Verification items for this drawing (mm, ordinates from the low corner). A direction names the side the tool comes from. Round coordinates to 2 decimals unless told otherwise and drop trailing zeros. Loops run counter-clockwise (first coordinate to the right, second up) from the corner with the lowest first, then second, coordinate; pieces in that order, holes last. Notation, with made-up numbers: (42, -17) - (51, -17) arc R5 cw to (51, -12) - close; hole circle Ø6 at (89, 81). An arc over 180 degrees is marked (long way). Put each result on its own line as item: value.
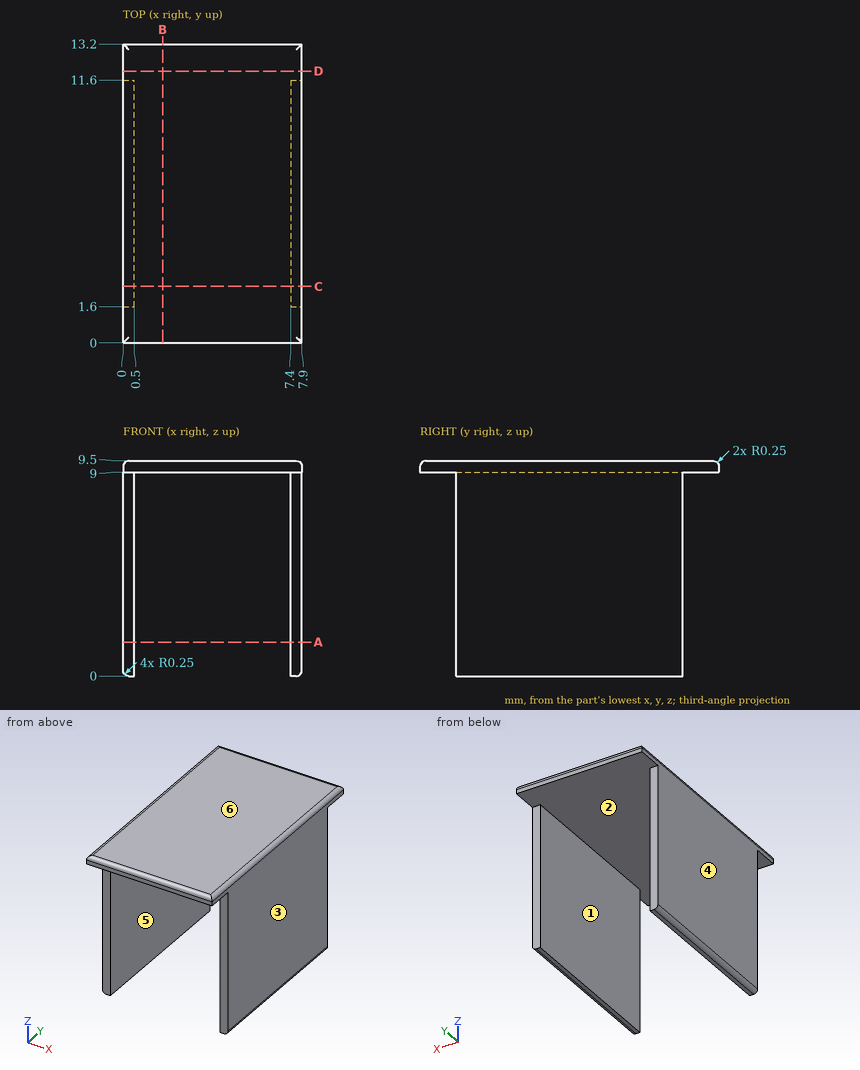
Item 1: Section check C-C on y = 2.5. Enter the section's corners in (x, z), then the cut area to 3 significant figures.
Filled sheet:
outline: (0, 0.25) arc R0.25 ccw to (0.25, 0) - (0.5, 0) - (0.5, 9) - (7.4, 9) - (7.4, 0) - (7.65, 0) arc R0.25 ccw to (7.9, 0.25) - (7.9, 9.25) arc R0.25 ccw to (7.65, 9.5) - (0.25, 9.5) arc R0.25 ccw to (0, 9.25) - close
area: 12.9 mm²
Item 2: Release check for a two-part mould opening along X. For the marked faces 1, 2, 3 and 4 record: +X half, -X half, draft (parallel to the pull), parting line (faces both ways), or undercut.
Filled sheet:
face 1: undercut
face 2: undercut
face 3: +X half
face 4: -X half
Item 3: Section check A-A on z = 1.5. Enter the section's corners in (x, y), then the cut area to 3 significant figures.
Filled sheet:
outline: (0, 1.6) - (0.5, 1.6) - (0.5, 11.6) - (0, 11.6) - close; (7.4, 1.6) - (7.9, 1.6) - (7.9, 11.6) - (7.4, 11.6) - close
area: 10.0 mm²
Item 4: Tool access check on the marked faces 5 and 6. Record the directions out of +Z, -Z, +X, -X, +Y, -Y that give a thin tool (end or side, any length) a straight path to the whole face; none if there is none.
Filled sheet:
face 5: -Z, +Y, -Y
face 6: +Z, +X, -X, +Y, -Y
Item 5: Go/stop test with a flat-tipped pin: pin 1 (0.6 mm diameter, centred on x = 0.5, z = 3.5, fed in from +Y). Record where the tip stops, or that it passes through.
Filled sheet:
pin 1: y = 11.6
Item 6: Section check B-B on x = 1.75. Enter the section's corners in (y, z), then the cut area to 3 significant figures.
Filled sheet:
outline: (0, 9) - (13.2, 9) - (13.2, 9.25) arc R0.25 ccw to (12.95, 9.5) - (0.25, 9.5) arc R0.25 ccw to (0, 9.25) - close
area: 6.57 mm²
Item 7: Section check D-D on y = 12. Enter the section's corners in (x, z), then the cut area to 3 significant figures.
Filled sheet:
outline: (0, 9) - (7.9, 9) - (7.9, 9.25) arc R0.25 ccw to (7.65, 9.5) - (0.25, 9.5) arc R0.25 ccw to (0, 9.25) - close
area: 3.92 mm²
Item 8: Thickness scan on line 1 (X direction, y = 8.5, z = 6); line 2 (Z direction, x = 3, y = 4); line 3 (Z direction, x = 7.75, y = 7). Record the ranges inside material, lowest first. Write a range as from..to.
Filled sheet:
line 1: 0..0.5, 7.4..7.9
line 2: 9..9.5
line 3: 0.02..9.48
